Geometry: final body of the model. Coordinates: model frame, mm. Face numbers are marked on the shaded views. Round coordinates to 2 decimals unless told otherwise and drop trailing zeros. Write each loop counter-clockwise with the first axis right and the second up, starting at its lowest first coordinate (ties: lowest second). Pieces come first, ordered by that corner, then holes.
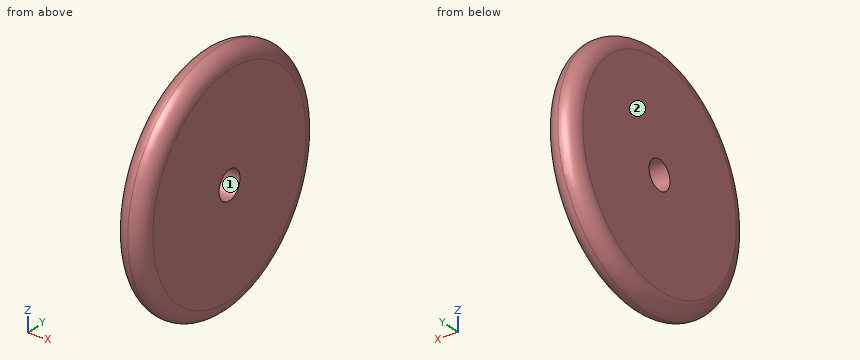
from build123d import *

# Parameters (mm, degrees)
SKETCH1_R           = 125
BOSS_EXTRUDE1_DEPTH = 30
FILLET1_R           = 15
SKETCH2_R           = 15
CUT_EXTRUDE1_DEPTH  = 180.30421084


with BuildPart() as part:
    # Sketch1 → Boss-Extrude1 (new body)
    with BuildSketch(Plane(origin=(0, 0, 0), x_dir=(0, 0, -1), z_dir=(1, 0, 0))):
        Circle(SKETCH1_R)
    extrude(amount=BOSS_EXTRUDE1_DEPTH)

    # Fillet1
    fillet1_edges = [part.edges().sort_by_distance(p)[0] for p in [
        (0, 0, 125),
        (30, 0, 125),
    ]]
    fillet(fillet1_edges, radius=FILLET1_R - 0.0001)  # a hair under: the kernel refuses the full size

    # Sketch2 → Cut-Extrude1 (cut, through all)
    with BuildSketch(Plane(origin=(30, 0, 0), x_dir=(0, 0, -1), z_dir=(1, 0, 0))):
        Circle(SKETCH2_R)
    extrude(amount=-CUT_EXTRUDE1_DEPTH, mode=Mode.SUBTRACT)


solid = part.part
1) Section D-D on x = 25.25. Output: boundary loops of the cut face in (y, z).
2) Line query: probe 1 along Y at (x, z) = (7.75, 0); probe 2 along Y at (x, z) = (17.25, 0); probe 3 along Y at (x, z) = (25.25, 105.5). Output: solid intervals per line, ascending.
3) Draft query along Y for the marked faces 1 and 2. Return one class per face: pulls with the +Y half, pulls with the -Y half, needs draft (parallel to the pull), parting line crosses it, or undercut.
4) First-contact query: P1, Ø8, axis at x = 9, y = -5, coming from the -Z side; P2, Ø1.5, axis at x = 15, y = 48.5, coming from the -Z side; P3, Ø1, axis at x = 9.5, z = 86.5, coming from the -Y side. Flat tips, straight axial feed; report the tip coordinate or a pass-through.
5) Section C-C on x = 11. Output: boundary loops of the cut face in (y, z).
Filled in:
1. outline: circle Ø241.9 at (0, 0); hole circle Ø30 at (0, 0)
2. probe 1: y = -123.13 to -15, 15 to 123.13
2. probe 2: y = -124.83 to -15, 15 to 124.83
2. probe 3: y = -59.15 to 59.15
3. face 1: undercut
3. face 2: needs draft
4. P1: stops at z = -124.78
4. P2: stops at z = -115.52
4. P3: stops at y = -89.34
5. outline: circle Ø248.91 at (0, 0); hole circle Ø30 at (0, 0)
